from build123d import *

# Parameters (mm, degrees)
F1_DEPTH = 7.5
F2_DEPTH = 10
F3_DEPTH = 8
F4_W     = 1.9
F4_H     = 2.2
F5_DEPTH = 3.801
F6_START = 1.7
F4_W_2   = 5
F4_H_2   = 11.4
F6_DEPTH = 2.101
F7_START = 3
F4_W_3   = 0.5
F7_DEPTH = 0.8
F8_DEPTH = 25


with BuildPart() as f1:
    # F0 (on Front) → F1 (new body, symmetric)
    with BuildSketch(Plane.XZ):
        with BuildLine():
            ThreePointArc((1.9, 1.9), (1.3435028843, 0.5564971157), (0, 0))
            Line((0, 0), (23.1, 0))
            ThreePointArc((23.1, 0), (21.9870057685, 2.6870057685), (19.3, 3.8))
            Line((19.3, 3.8), (0, 3.8))
            ThreePointArc((0, 3.8), (1.3435028843, 3.2435028843), (1.9, 1.9))
        make_face()
        with BuildLine():
            ThreePointArc((-1.7853571071, 1.25), (-1.0897247359, 0.3435617584), (0, 0))
            ThreePointArc((0, 0), (1.3435028843, 0.5564971157), (1.9, 1.9))
            ThreePointArc((1.9, 1.9), (1.3435028843, 3.2435028843), (0, 3.8))
            ThreePointArc((0, 3.8), (-1.0897247359, 3.4564382416), (-1.7853571071, 2.55))
            Line((-1.7853571071, 2.55), (-0.8874119675, 2.55))
            ThreePointArc((-0.8874119675, 2.55), (0.3419406643, 2.9455030283), (1.1, 1.9))
            ThreePointArc((1.1, 1.9), (0.3419406643, 0.8544969717), (-0.8874119675, 1.25))
            Line((-0.8874119675, 1.25), (-1.7853571071, 1.25))
        make_face()
        with BuildLine():
            ThreePointArc((-1.7853571071, 2.55), (-1.9, 1.9), (-1.7853571071, 1.25))
            Line((-1.7853571071, 1.25), (-0.8874119675, 1.25))
            ThreePointArc((-0.8874119675, 1.25), (-1.1, 1.9), (-0.8874119675, 2.55))
            Line((-0.8874119675, 2.55), (-1.7853571071, 2.55))
        make_face()
    extrude(amount=F1_DEPTH, both=True)

    # F0 (on Front) → F2 (join, symmetric)
    with BuildSketch(Plane.XZ):
        with BuildLine():
            ThreePointArc((-0.8874119675, 2.55), (-1.1, 1.9), (-0.8874119675, 1.25))
            ThreePointArc((-0.8874119675, 1.25), (0.3419406643, 0.8544969717), (1.1, 1.9))
            ThreePointArc((1.1, 1.9), (0.3419406643, 2.9455030283), (-0.8874119675, 2.55))
        make_face()
    extrude(amount=F2_DEPTH, both=True)

    # F0 (on Front) → F3 (join, symmetric)
    with BuildSketch(Plane.XZ):
        with BuildLine():
            ThreePointArc((-1.7853571071, 2.55), (-1.9, 1.9), (-1.7853571071, 1.25))
            Line((-1.7853571071, 1.25), (-0.8874119675, 1.25))
            ThreePointArc((-0.8874119675, 1.25), (-1.1, 1.9), (-0.8874119675, 2.55))
            Line((-0.8874119675, 2.55), (-1.7853571071, 2.55))
        make_face()
    extrude(amount=F3_DEPTH, both=True)

    # F4 (on Top) → F5 (cut, through all)
    with BuildSketch(Plane.XY):
        with Locations((-0.95, 4.6)):
            Rectangle(F4_W, F4_H)
        with BuildLine():
            Line((0, 5.7), (0, 3.5))
            Line((0, 3.5), (7, 3.5))
            ThreePointArc((7, 3.5), (8.1, 4.6), (7, 5.7))
            Line((7, 5.7), (0, 5.7))
        make_face()
        with Locations((-0.95, -4.6)):
            Rectangle(F4_W, F4_H)
        with BuildLine():
            Line((0, -3.5), (0, -5.7))
            Line((0, -5.7), (7, -5.7))
            ThreePointArc((7, -5.7), (8.1, -4.6), (7, -3.5))
            Line((7, -3.5), (0, -3.5))
        make_face()
    extrude(amount=F5_DEPTH, mode=Mode.SUBTRACT)

    # F4 (on Top) → F6 (cut)
    with BuildSketch(Plane.XY.offset(F6_START)):
        with BuildLine():
            ThreePointArc((7, -3.5), (8.1, -4.6), (7, -5.7))
            Line((7, -5.7), (17.6, -5.7))
            Line((17.6, -5.7), (17.6, 5.7))
            Line((17.6, 5.7), (7, 5.7))
            ThreePointArc((7, 5.7), (8.1, 4.6), (7, 3.5))
            Line((7, 3.5), (0, 3.5))
            Line((0, 3.5), (0, -3.5))
            Line((0, -3.5), (7, -3.5))
        make_face()
        with Locations((20.6, 0)):
            Rectangle(F4_W_2, F4_H_2)
    extrude(amount=F6_DEPTH, mode=Mode.SUBTRACT)

    # F4 (on Top) → F7 (cut)
    with BuildSketch(Plane.XY.offset(F7_START)):
        with Locations((17.85, 0)):
            Rectangle(F4_W_3, F4_H_2)
    extrude(amount=F7_DEPTH, mode=Mode.SUBTRACT)

    # F4 (on Top) → F8 (cut)
    with BuildSketch(Plane.XY):
        Polygon((-1.1, 8.9), (0, 10), (-1.1, 10), align=None)
        Polygon((0, -10), (-1.1, -8.9), (-1.1, -10), align=None)
    extrude(amount=F8_DEPTH, mode=Mode.SUBTRACT)


solid = f1.part
Source: CAD feature listing. Evaluate the final solid. Frame: model axes, mm. A direction names the side the tool comes from. Give positions to 0.01 mm unless a question says otherwise; leave off trailing zeros. Write each loop counter-clockwise with the first axis right and the second up, starting at its lowest first coordinate (ties: lowest second). Pieces come first, ordered by that corner, then holes. Notation, with made-up numbers: (23.25, 51.5) -> (36.25, 51.5) arc R16 ccw to (36.25, 68.5) -> close; hole circle Ø1 at (80.25, -37.75). An arc over 180 degrees is marked (long way). Write item = value, one per line.
Q1. Cut plane D-D on z = 0.35. Return loops of the section in (x, y).
Here are the results:
outline = (-1.1, -7.5) -> (23.08, -7.5) -> (23.08, 7.5) -> (-1.1, 7.5) -> (-1.1, 5.7) -> (7, 5.7) arc R1.1 cw to (7, 3.5) -> (-1.1, 3.5) -> (-1.1, -3.5) -> (7, -3.5) arc R1.1 cw to (7, -5.7) -> (-1.1, -5.7) -> close
Q2. Reachability of faces 1 (the face through (11, 0, 1.7)), 2 (the face through (2, -3.5, 1)), 3 (the face through (20, 0, 1.7)) from +Z, -Z, +X, -X, +Y, -Y: full face, straight path, thin tool, end or side. Return the list, or none.
Here are the results:
face_1 = +Z
face_2 = +Z, -Z, -X
face_3 = +Z, +X
Q3. Line query: line 1 (Y direction, x = 6.75, z = 1.3); line 2 (Y direction, x = 14.75, z = 2.5); line 3 (Y direction, x = 8, z = 1.15). Output: solid intervals per line, ascending. Write a range as from..to.
Here are the results:
line_1 = -7.5..-5.7, -3.5..3.5, 5.7..7.5
line_2 = -7.5..-5.7, 5.7..7.5
line_3 = -7.5..-5.06, -4.14..4.14, 5.06..7.5
Q4. Cut plane B-B on y = 4.6. Return loops of the section in (x, z).
Here are the results:
outline = (8.1, 0) -> (23.1, 0) arc R3.8 ccw to (22.7, 1.7) -> (18.1, 1.7) -> (18.1, 3) -> (17.6, 3) -> (17.6, 1.7) -> (8.1, 1.7) -> close
Q5. First-contact query: pin 1 (1.5 mm diameter, centred on x = 7, z = 1, fed in from +Y); pin 2 (1 mm diameter, centred on y = -1, z = 3, fed in from +X); pin 3 (5.5 mm diameter, centred on x = 11.5, y = -2.5, fed in from +Z). Flat tips, straight axial feed; report the tip coordinate or a pass-through.
Here are the results:
pin_1 = 7.5
pin_2 = 18.1
pin_3 = 1.7
Q6. Mould query, pull axis X, two halves, no side actions, for faces 4 (the face through (0, 0, 3)), 5 (the face through (17.6, 0, 2)), 6 (the face through (8.1, 4.6, 0.8)), 7 (the face through (11, 0, 0)). Classes: +X half, -X half, draft (parallel to the pull), parting line (faces both ways), or undercut.
Here are the results:
face_4 = undercut
face_5 = undercut
face_6 = -X half
face_7 = draft
Q7. Cut plane C-C on x = 11. Return loops of the section in (y, z).
Here are the results:
outline = (-7.5, 0) -> (7.5, 0) -> (7.5, 3.8) -> (5.7, 3.8) -> (5.7, 1.7) -> (-5.7, 1.7) -> (-5.7, 3.8) -> (-7.5, 3.8) -> close
Q8. Cut plane A-A on x = 2.25. Return loops of the section in (y, z), then the cut area to 3 significant figures.
Here are the results:
outline = (-7.5, 0) -> (-5.7, 0) -> (-5.7, 3.8) -> (-7.5, 3.8) -> close; (-3.5, 0) -> (3.5, 0) -> (3.5, 1.7) -> (-3.5, 1.7) -> close; (5.7, 0) -> (7.5, 0) -> (7.5, 3.8) -> (5.7, 3.8) -> close
area = 25.6 mm²
